Read the model definition and answer for the solid it produces. Units are mm, in the model's axes. A direction names the side the tool comes from. Coordinates: 2 decimals unless noted, no trailing zeros. Write each loop counter-clockwise with the first axis right and the second up, starting at its lowest first coordinate (ties: lowest second). Pieces come first, ordered by that corner, then holes. Notation, with made-up numbers: (-17, 85) -> (-6, 85) arc R29 ccw to (-6, 120) -> close; hole circle Ø5 at (27.25, 55). An arc over 180 degrees is marked (long way). One line per item, written item: value. Start each with the question number.
1. Consider line 1 along X through (y, z) = (1.45, 0); line 2 along X through (y, z) = (2, -5); line 3 along X through (y, z) = (1.05, 13). Determine where each line is inside the solid, lowest interval first.
2. Find section A-A, the plane x = -15. Write down the section's boundary in (y, z), and give its area (3 significant figures).
3. Given P1, Ø1.5, axis at x = 14, z = 1.5, coming from the -Y side, flat-ended and moving along its own axis, determine where the tip first touches the part or whether it passes through.
4. For faces 4 (the flat face through (-23, 1, 8)), 5 (the cylindrical face through (-13.1, 1.48, 7.54)), determine the directions among +Z, -Z, +X, -X, +Y, -Y from which every point of the face is accessible in a straight line to the end or side of a thin tool.
5. Find section D-D, the plane y = 1.7. State how many separate pieces and enclosed holes the cut face has, and give its area (3 significant figures).
6. Find section C-C, the plane x = 0. Write down the section's boundary in (y, z).
7. Find section B-B, the plane z = 12.5. Write down the section's boundary in (x, y).
8. For a pull along X with two mould halves and no side action, classify faces 1 (the cylindrical face through (11.36, 1.52, 1.89)), 2 (the flat face through (0, 3, 4)), 3 (the cylindrical face through (-22.14, 1.52, -7.1)) as pulls with the +X half, pulls with the -X half, needs draft (parallel to the pull), parting line crosses it, or undercut.
```python
from build123d import *

# Parameters (mm, degrees)
SKETCH_4_W          = 46
SKETCH_4_H          = 16
EXTRUDE_3_DEPTH     = 3
CUT_EXTRUDE_1_REACH = 26.536
SKETCH_5_R          = 4.1
SKETCH_6_W          = 46
SKETCH_6_H          = 3
EXTRUDE_4_DEPTH     = 16
CUT_EXTRUDE_2_REACH = 35.377
SKETCH_9_R          = 1.6
CUT_EXTRUDE_4_REACH = 35.377
SKETCH_11_R         = 1.15
SKETCH_11_R_2       = 2.1
CUT_EXTRUDE_5_REACH = 35.377
SKETCH_12_W         = 28
SKETCH_12_H         = 12
FILLET_3_R          = 3


with BuildPart() as part:
    # 草图4 → 凸台-拉伸3 (new body)
    with BuildSketch(Plane(origin=(0, 0, 0), x_dir=(1, 0, 0), z_dir=(0, 1, 0))):
        Rectangle(SKETCH_4_W, SKETCH_4_H)
    extrude(amount=EXTRUDE_3_DEPTH)

    # 草图5 → 切除-拉伸1 (cut, up to next)
    with BuildSketch(Plane(origin=(0, 3, 0), x_dir=(1, 0, 0), z_dir=(0, 1, 0)), mode=Mode.PRIVATE) as cut_extrude_1_sk1:
        with Locations(Location((-15, 0, 0), (0, 0, 270))):
            Circle(SKETCH_5_R)
    cut_extrude_1_tool1 = extrude(cut_extrude_1_sk1.sketch, amount=-CUT_EXTRUDE_1_REACH, mode=Mode.PRIVATE) & part.part
    # 草图5 → 切除-拉伸1 (cut, up to next)
    with BuildSketch(Plane(origin=(0, 3, 0), x_dir=(1, 0, 0), z_dir=(0, 1, 0)), mode=Mode.PRIVATE) as cut_extrude_1_sk2:
        with Locations(Location((15, 0, 0), (0, 0, 270))):
            Circle(SKETCH_5_R)
    cut_extrude_1_tool2 = extrude(cut_extrude_1_sk2.sketch, amount=-CUT_EXTRUDE_1_REACH, mode=Mode.PRIVATE) & part.part
    add(cut_extrude_1_tool1.solids().sort_by_distance((-15, 3, 0))[0], mode=Mode.SUBTRACT)
    add(cut_extrude_1_tool2.solids().sort_by_distance((15, 3, 0))[0], mode=Mode.SUBTRACT)

    # 草图6 → 凸台-拉伸4 (add)
    with BuildSketch(Plane.XY.offset(8)):
        with Locations((0, 1.5)):
            Rectangle(SKETCH_6_W, SKETCH_6_H)
    extrude(amount=EXTRUDE_4_DEPTH)

    # 草图9 → 切除-拉伸2 (cut, up to next)
    with BuildSketch(Plane(origin=(0, 3, 0), x_dir=(1, 0, 0), z_dir=(0, 1, 0)), mode=Mode.PRIVATE) as cut_extrude_2_sk1:
        with Locations(Location((-19, -18, 0), (0, 0, 270))):
            Circle(SKETCH_9_R)
    cut_extrude_2_tool1 = extrude(cut_extrude_2_sk1.sketch, amount=-CUT_EXTRUDE_2_REACH, mode=Mode.PRIVATE) & part.part
    # 草图9 → 切除-拉伸2 (cut, up to next)
    with BuildSketch(Plane(origin=(0, 3, 0), x_dir=(1, 0, 0), z_dir=(0, 1, 0)), mode=Mode.PRIVATE) as cut_extrude_2_sk2:
        with Locations(Location((19, -18, 0), (0, 0, 270))):
            Circle(SKETCH_9_R)
    cut_extrude_2_tool2 = extrude(cut_extrude_2_sk2.sketch, amount=-CUT_EXTRUDE_2_REACH, mode=Mode.PRIVATE) & part.part
    add(cut_extrude_2_tool1.solids().sort_by_distance((-19, 3, 18))[0], mode=Mode.SUBTRACT)
    add(cut_extrude_2_tool2.solids().sort_by_distance((19, 3, 18))[0], mode=Mode.SUBTRACT)

    # 草图11 → 切除-拉伸4 (cut, up to next)
    with BuildSketch(Plane(origin=(0, 3, 0), x_dir=(1, 0, 0), z_dir=(0, 1, 0)), mode=Mode.PRIVATE) as cut_extrude_4_sk1:
        with Locations(Location((-11, 5, 0), (0, 0, 270))):
            Circle(SKETCH_11_R)
    cut_extrude_4_tool1 = extrude(cut_extrude_4_sk1.sketch, amount=-CUT_EXTRUDE_4_REACH, mode=Mode.PRIVATE) & part.part
    # 草图11 → 切除-拉伸4 (cut, up to next)
    with BuildSketch(Plane(origin=(0, 3, 0), x_dir=(1, 0, 0), z_dir=(0, 1, 0)), mode=Mode.PRIVATE) as cut_extrude_4_sk2:
        with Locations(Location((11, 5, 0), (0, 0, 270))):
            Circle(SKETCH_11_R)
    cut_extrude_4_tool2 = extrude(cut_extrude_4_sk2.sketch, amount=-CUT_EXTRUDE_4_REACH, mode=Mode.PRIVATE) & part.part
    # 草图11 → 切除-拉伸4 (cut, up to next)
    with BuildSketch(Plane(origin=(0, 3, 0), x_dir=(1, 0, 0), z_dir=(0, 1, 0)), mode=Mode.PRIVATE) as cut_extrude_4_sk3:
        with Locations(Location((0, 5, 0), (0, 0, 270))):
            Circle(SKETCH_11_R_2)
    cut_extrude_4_tool3 = extrude(cut_extrude_4_sk3.sketch, amount=-CUT_EXTRUDE_4_REACH, mode=Mode.PRIVATE) & part.part
    add(cut_extrude_4_tool1.solids().sort_by_distance((-11, 3, -5))[0], mode=Mode.SUBTRACT)
    add(cut_extrude_4_tool2.solids().sort_by_distance((11, 3, -5))[0], mode=Mode.SUBTRACT)
    add(cut_extrude_4_tool3.solids().sort_by_distance((0, 3, -5))[0], mode=Mode.SUBTRACT)

    # 草图12 → 切除-拉伸5 (cut, up to next)
    with BuildSketch(Plane(origin=(0, 3, 0), x_dir=(1, 0, 0), z_dir=(0, 1, 0)), mode=Mode.PRIVATE) as cut_extrude_5_sk1:
        with Locations((0, -12.680818863)):
            Rectangle(SKETCH_12_W, SKETCH_12_H)
    cut_extrude_5_tool1 = extrude(cut_extrude_5_sk1.sketch, amount=-CUT_EXTRUDE_5_REACH, mode=Mode.PRIVATE) & part.part
    add(cut_extrude_5_tool1.solids().sort_by_distance((0, 3, 12.680819))[0], mode=Mode.SUBTRACT)

    # 圆角3
    fillet_3_edges = [part.edges().sort_by_distance(p)[0] for p in [
        (-23, 1.5, 24),
        (23, 1.5, 24),
        (14, 1.5, 6.680818863),
        (14, 1.5, 18.680818863),
        (-14, 1.5, 18.680818863),
        (-14, 1.5, 6.680818863),
        (-23, 1.5, -8),
        (23, 1.5, -8),
    ]]
    fillet(fillet_3_edges, radius=FILLET_3_R)


solid = part.part
```
Answer block:
1. line 1: x = -23 to -19.1, -10.9 to 10.9, 19.1 to 23
1. line 2: x = -23 to -12.15, -9.85 to -2.1, 2.1 to 9.85, 12.15 to 23
1. line 3: x = -23 to -14, 14 to 23
2. outline: (0, -8) -> (3, -8) -> (3, -4.1) -> (0, -4.1) -> close; (0, 4.1) -> (3, 4.1) -> (3, 24) -> (0, 24) -> close
2. area: 71.4 mm2
3. P1: passes through
4. face 4: +Z, -Z, -X, +Y, -Y
4. face 5: +Y, -Y
5. separate pieces: 1
5. enclosed holes: 8
5. area: 992 mm2
6. outline: (0, -8) -> (3, -8) -> (3, -7.1) -> (0, -7.1) -> close; (0, -2.9) -> (3, -2.9) -> (3, 6.68) -> (0, 6.68) -> close; (0, 18.68) -> (3, 18.68) -> (3, 24) -> (0, 24) -> close
7. outline: (-23, 0) -> (-14, 0) -> (-14, 3) -> (-23, 3) -> close; (14, 0) -> (23, 0) -> (23, 3) -> (14, 3) -> close
8. face 1: undercut
8. face 2: needs draft
8. face 3: pulls with the -X half
